Geometry check sheet. Reference: the model listing, model coordinates, mm. A direction names the side the tool comes from. Give positions to 0.01 mm unless a question says otherwise; leave off trailing zeros. Loops run counter-clockwise (first coordinate to the right, second up) from the corner with the lowest first, then second, coordinate; pieces in that order, holes last. Notation, with made-up numbers: (-20.75, 40.25) - (-6.75, 40.25) arc R13 cw to (-6.75, 50.25) - close; hole circle Ø5 at (65, -31). An arc over 180 degrees is marked (long way). Write item = value, one per line. Start each with the question number.
from build123d import *

# Parameters (mm, degrees)
SKETCH1_R           = 2.3
EXTRUDE1_DEPTH      = 1
SKETCH2_W           = 12
SKETCH2_H           = 5
EXTRUDE2_DEPTH      = 3.8
SKETCH3_W           = 5
SKETCH3_H           = 3.8
EXTRUDE3_DEPTH      = 1.5
SKETCH4_W           = 6
SKETCH4_H           = 7.1
EXTRUDE4_DEPTH      = 2
EXTRUDE5_DEPTH      = 26.91110545
EXTRUDE5_DEPTH_BACK = 26.91110545
SKETCH5_R           = 1
SKETCH6_R           = 0.5
EXTRUDE6_DEPTH      = 27.076529402


with BuildPart() as part:
    # Sketch1 → Extrude1 (new body)
    with BuildSketch(Plane(origin=(0, 0, 0), x_dir=(1, 0, 0), z_dir=(0, 1, 0))):
        with BuildLine():
            Line((-7.1, 18.3), (-7.1, 16.866534914))
            ThreePointArc((-7.1, 16.866534914), (-14.175345058, 11.573659425), (-17.945901639, 3.582543001))
            ThreePointArc((-17.945901639, 3.582543001), (-14.7, 0), (-17.945901639, -3.582543001))
            ThreePointArc((-17.945901639, -3.582543001), (-13.830201246, -11.983969855), (-6.1, -17.253405461))
            Line((-6.1, -17.253405461), (-6.1, -18.3))
            Line((-6.1, -18.3), (6.1, -18.3))
            Line((6.1, -18.3), (6.1, -17.253405461))
            ThreePointArc((6.1, -17.253405461), (13.830201246, -11.983969855), (17.945901639, -3.582543001))
            ThreePointArc((17.945901639, -3.582543001), (14.7, 0), (17.945901639, 3.582543001))
            ThreePointArc((17.945901639, 3.582543001), (14.175345058, 11.573659425), (7.1, 16.866534914))
            Line((7.1, 16.866534914), (7.1, 18.3))
            Line((7.1, 18.3), (-7.1, 18.3))
        make_face()
        with Locations(Location((-10, 10, 0), (0, 0, 270))):
            Circle(SKETCH1_R, mode=Mode.SUBTRACT)
        with Locations(Location((10, 10, 0), (0, 0, 270))):
            Circle(SKETCH1_R, mode=Mode.SUBTRACT)
        with Locations(Location((10, -10, 0), (0, 0, 270))):
            Circle(SKETCH1_R, mode=Mode.SUBTRACT)
        with Locations(Location((-10, -10, 0), (0, 0, 270))):
            Circle(SKETCH1_R, mode=Mode.SUBTRACT)
    extrude(amount=EXTRUDE1_DEPTH)

    # Sketch2 → Extrude2 (add)
    with BuildSketch(Plane(origin=(0, 1, 0), x_dir=(1, 0, 0), z_dir=(0, 1, 0))):
        with Locations((0, 15.8)):
            Rectangle(SKETCH2_W, SKETCH2_H)
    extrude(amount=EXTRUDE2_DEPTH)

    # Sketch3 → Extrude3 (add)
    with BuildSketch(Plane(origin=(0, 1, 0), x_dir=(1, 0, 0), z_dir=(0, 1, 0))):
        Rectangle(SKETCH3_W, SKETCH3_H)
    extrude(amount=EXTRUDE3_DEPTH)

    # Sketch4 → Extrude4 (add)
    with BuildSketch(Plane.XZ):
        with Locations((0, 8.25)):
            Rectangle(SKETCH4_W, SKETCH4_H)
    extrude(amount=EXTRUDE4_DEPTH)

    # Sketch5 → Extrude5 (cut, two sides: drawn at the far end of the back side and taken through both)
    with BuildSketch(Plane(origin=(0, 1, 0), x_dir=(1, 0, 0), z_dir=(0, 1, 0)).offset(-EXTRUDE5_DEPTH_BACK)):
        with Locations(Location((-8.9, 14.15, 0), (0, 0, 270))):
            Circle(SKETCH5_R)
        with Locations(Location((8.9, -14.15, 0), (0, 0, 270))):
            Circle(SKETCH5_R)
    extrude(amount=EXTRUDE5_DEPTH + EXTRUDE5_DEPTH_BACK, mode=Mode.SUBTRACT)

    # Sketch6 → Extrude6 (cut, through all)
    with BuildSketch(Plane.XZ):
        with Locations(Location((-13.3, 0, 0), (0, 0, 270))):
            Circle(SKETCH6_R)
        with Locations(Location((-14.764466094, 3.535533906, 0), (0, 0, 270))):
            Circle(SKETCH6_R)
        with Locations(Location((-14.764466094, -3.535533906, 0), (0, 0, 270))):
            Circle(SKETCH6_R)
    extrude(amount=-EXTRUDE6_DEPTH, mode=Mode.SUBTRACT)


solid = part.part
1) Cross-section at B-B on x = 8.9. Enter the section's corners in (y, z), and give its area (3 significant figures).
2) Cross-section at A-A on z = 11. Enter the section's corners in (x, y).
3) Cross-section at D-D on x = -13.3. Enter the section's corners in (y, z).
4) Gauge pin test, flat ends, axial feed: P1, Ø4, axis at x = -7, z = 9, coming from the +Y side; P2, Ø1.9, axis at x = 0, z = -1, coming from the +Y side; P3, Ø1, axis at y = -1, z = 7, coming from the -X side; P4, Ø3, axis at x = 10, z = 10, coming from the -Y side. Record the tip position at first contact, or that the pin passes through.
5) Tool access check on faces 4 (the face through (-6.1, 0.5, 17.8)), 5 (the face through (0, 3, -13.3)), 6 (the face through (6.1, 0.5, 17.8)), 7 (the face through (7.1, 0.5, -17.6)). Record the directions out of +Z, -Z, +X, -X, +Y, -Y that give a thin tool (end or side, any length) a straight path to the whole face; none if there is none.
6) Material ranges on line 1 along X through (y, z) = (0.4, 0); line 2 along Z through (x, y) = (-8.9, 0.35); line 3 along X through (y, z) = (0.4, 10), recorded low to high.
7) Release check for a two-part mould opening along Z. For faces 1 (the face through (0, 4.8, -16)), 2 (the face through (0, -1, 4.7)), 3 (the face through (-8.45, 0.49, -11.7)) record: pulls with the +Z half, pulls with the -Z half, needs draft (parallel to the pull), parting line crosses it, or undercut.
8) Cross-section at C-C on y = 0.5. Give the number of separate pieces and of enclosed holes in the cut face, and give its area (3 significant figures).
Checked values:
q1.outline = (0, -15.99) - (1, -15.99) - (1, -12.02) - (0, -12.02) - close; (0, -7.98) - (1, -7.98) - (1, 7.98) - (0, 7.98) - close; (0, 12.02) - (1, 12.02) - (1, 13.15) - (0, 13.15) - close; (0, 15.15) - (1, 15.15) - (1, 15.99) - (0, 15.99) - close
q1.area = 21.9 mm²
q2.outline = (-14.62, 0) - (-12.07, 0) - (-12.07, 1) - (-14.62, 1) - close; (-7.93, 0) - (-3, 0) - (-3, -2) - (3, -2) - (3, 0) - (7.93, 0) - (7.93, 1) - (-7.93, 1) - close; (12.07, 0) - (14.62, 0) - (14.62, 1) - (12.07, 1) - close
q3.outline = (0, -12.57) - (1, -12.57) - (1, -0.5) - (0, -0.5) - close; (0, 0.5) - (1, 0.5) - (1, 12.57) - (0, 12.57) - close
q4.P1 = 1
q4.P2 = 2.5
q4.P3 = -3
q4.P4 = through
q5.face_4 = +Z, -X, +Y, -Y
q5.face_5 = +X, -X, +Y
q5.face_6 = +Z, +X, +Y, -Y
q5.face_7 = -Z, +X, +Y, -Y
q6.line_1 = -14.7 to -13.8, -12.8 to 14.7
q6.line_2 = -15.99 to -15.15, -13.15 to -12.02, -7.98 to 7.98, 12.02 to 15.99
q6.line_3 = -15.33 to -12.3, -7.7 to 7.7, 12.3 to 15.33
q7.face_1 = needs draft
q7.face_2 = pulls with the -Z half
q7.face_3 = undercut
q8.separate_pieces = 1
q8.enclosed_holes = 9
q8.area = 949 mm²
